Here's how the part is built. I have some questions about the finished solid (model axes, mm). A direction names the side the tool comes from. Give positions to 0.01 mm unless a question says otherwise; leave off trailing zeros. Write each loop counter-clockwise with the first axis right and the second up, starting at its lowest first coordinate (ties: lowest second). Pieces come first, ordered by that corner, then holes. Notation, with made-up numbers: (72.5, 38.25) -> (100.5, 38.25) arc R14 cw to (100.5, 48.25) -> close; hole circle Ø11 at (-18.5, -23). An arc over 180 degrees is marked (long way). Return JSON: item names as keys, results as strings.
from build123d import *

# Parameters (mm, degrees)
SKETCH1_R           = 1
SKETCH1_R_2         = 4
BOSS_EXTRUDE1_DEPTH = 3
SKETCH2_W           = 2.5
SKETCH2_H           = 22
BOSS_EXTRUDE2_DEPTH = 16
SKETCH3_R           = 1.132393425
SKETCH3_R_2         = 1.130977438
CUT_EXTRUDE1_DEPTH  = 6


with BuildPart() as part:
    # Sketch1 → Boss-Extrude1 (new body)
    with BuildSketch(Plane(origin=(0, 0, 0), x_dir=(1, 0, 0), z_dir=(0, 1, 0))):
        with BuildLine():
            Line((-14, -11), (-14, 11))
            Line((-14, 11), (6, 11))
            ThreePointArc((6, 11), (17, 0), (6, -11))
            Line((6, -11), (-14, -11))
        make_face()
        with Locations((6, -7)):
            Circle(SKETCH1_R, mode=Mode.SUBTRACT)
        with Locations((-1, 0)):
            Circle(SKETCH1_R, mode=Mode.SUBTRACT)
        with Locations((6, 0)):
            Circle(SKETCH1_R_2, mode=Mode.SUBTRACT)
        with Locations((13, 0)):
            Circle(SKETCH1_R, mode=Mode.SUBTRACT)
        with Locations((6, 7)):
            Circle(SKETCH1_R, mode=Mode.SUBTRACT)
    extrude(amount=BOSS_EXTRUDE1_DEPTH)

    # Sketch2 → Boss-Extrude2 (add)
    with BuildSketch(Plane(origin=(0, 3, 0), x_dir=(1, 0, 0), z_dir=(0, 1, 0))):
        with Locations((-12.75, 0)):
            Rectangle(SKETCH2_W, SKETCH2_H)
    extrude(amount=BOSS_EXTRUDE2_DEPTH)

    # Sketch3 → Cut-Extrude1 (cut)
    with BuildSketch(Plane(origin=(-11.5, 0, 0), x_dir=(0, 0, -1), z_dir=(1, 0, 0))):
        with Locations((6.9, 16)):
            Circle(SKETCH3_R)
        with Locations((-6.9, 16)):
            Circle(SKETCH3_R_2)
    extrude(amount=-CUT_EXTRUDE1_DEPTH, mode=Mode.SUBTRACT)


solid = part.part
1. Suppose I cut it at D-D, the plane x = -4.5. List the corners of the cut face in (y, z) for me, and give its area (3 significant figures).
Taken from the geometry:
{"outline": "(0, -11) -> (3, -11) -> (3, 11) -> (0, 11) -> close", "area": "66.0 mm²"}
2. Suppose I cut it at B-B, the plane z = -7. List the corners of the cut face in (x, y) for me, and give its area (3 significant figures).
Taken from the geometry:
{"outline": "(-14, 0) -> (5, 0) -> (5, 3) -> (-11.5, 3) -> (-11.5, 14.87) -> (-14, 14.87) -> close; (-14, 17.13) -> (-11.5, 17.13) -> (-11.5, 19) -> (-14, 19) -> close; (7, 0) -> (14.49, 0) -> (14.49, 3) -> (7, 3) -> close", "area": "114 mm²"}
3. If I drill on line 1 (X direction, y = 0.7, z = 0); line 2 (Y direction, x = -12.8, z = -6.9); line 3 (Z direction, x = -1, y = 0.7), over which ranges is the centre line in solid material (lowest first)? Write a range as [from, to].
Taken from the geometry:
{"line 1": "x = [-14, -2], [0, 2], [10, 12], [14, 17]", "line 2": "y = [0, 14.87], [17.13, 19]", "line 3": "z = [-11, -1], [1, 11]"}
4. Suppose I cut it at C-C, the plane y = 14.25. List the corners of the cut face in (x, z) for me.
Taken from the geometry:
{"outline": "(-14, -11) -> (-11.5, -11) -> (-11.5, 11) -> (-14, 11) -> close"}
5. For pin 1 Ø2.5 at (x, z) = (-1, 0) entering from -Y; pin 2 Ø1.5 at (y, z) = (15, 6.5) entering from +X; pin 3 Ø2.5 at (x, z) = (6, -7) entering from +Y, each with a flat end and sliding along its axis, tell me the tip position at first contact or that it passes through.
Taken from the geometry:
{"pin 1": "stops at y = 0", "pin 2": "stops at x = -11.5", "pin 3": "stops at y = 3"}
6. Suppose I cut it at A-A, the plane x = -1. List the corners of the cut face in (y, z) for me.
Taken from the geometry:
{"outline": "(0, -11) -> (3, -11) -> (3, -1) -> (0, -1) -> close; (0, 1) -> (3, 1) -> (3, 11) -> (0, 11) -> close"}
7. If we mould it in two halves opening along X, with no side actions, what happens to faces 1 (the face through (-8, 2, 11)), 2 (the face through (5.133, 1.479, 3.905)), 3 (the face through (5.263, 1.479, -7.676)), 4 (the face through (17, 1, 0))? For each: released by +X, released by -X, zero draft, split by the parting line, or undercut.
Taken from the geometry:
{"face 1": "zero draft", "face 2": "undercut", "face 3": "undercut", "face 4": "released by +X"}
8. Which directions (+Z, -Z, +X, -X, +Y, -Y) give clear straight access to the entire face, cutting with the end or side of a thin tool? Please do faces 5 (the face through (-11.5, 11, 0)), 6 (the face through (1.7, 0, -0.2)).
Taken from the geometry:
{"face 5": "+Z, -Z, +X, +Y", "face 6": "+Z, -Z, +X, -X, -Y"}
